Work out the finished part from the listing and answer in its coordinate system (mm). A direction names the side the tool comes from. Round coordinates to 2 decimals unless told otherwise and drop trailing zeros. Loops run counter-clockwise (first coordinate to the right, second up) from the corner with the lowest first, then second, coordinate; pieces in that order, holes last.
```python
from build123d import *

# Parameters (mm, degrees)
SKETCH1_W           = 139
SKETCH1_H           = 62
SKETCH1_R           = 3.75
SKETCH1_R_2         = 1.65
SKETCH1_R_3         = 3.1
SKETCH1_W_2         = 2.2
SKETCH1_H_2         = 1.1
SKETCH1_W_3         = 2.7
SKETCH1_H_3         = 1.2
BOSS_EXTRUDE1_DEPTH = 3


with BuildPart() as part:
    # Sketch1 → Boss-Extrude1 (new body)
    with BuildSketch(Plane.XY):
        with Locations((69.5, 31)):
            Rectangle(SKETCH1_W, SKETCH1_H)
        with Locations((94.5, 10)):
            Circle(SKETCH1_R, mode=Mode.SUBTRACT)
        with Locations((4, 33)):
            Circle(SKETCH1_R_2, mode=Mode.SUBTRACT)
        with Locations((135, 33)):
            Circle(SKETCH1_R_2, mode=Mode.SUBTRACT)
        with Locations((135, 11)):
            Circle(SKETCH1_R_2, mode=Mode.SUBTRACT)
        with Locations((4, 11)):
            Circle(SKETCH1_R_2, mode=Mode.SUBTRACT)
        with Locations((106.75, 31.217622393)):
            Circle(SKETCH1_R, mode=Mode.SUBTRACT)
        with Locations((124, 21.5)):
            Circle(SKETCH1_R_2, mode=Mode.SUBTRACT)
        with Locations((44.5, 10)):
            Circle(SKETCH1_R, mode=Mode.SUBTRACT)
        with Locations(Location((15, 21.5, 0), (0, 0, 180))):
            Circle(SKETCH1_R_2, mode=Mode.SUBTRACT)
        with Locations((56.5, 52)):
            Circle(SKETCH1_R_3, mode=Mode.SUBTRACT)
        with Locations((4, 55)):
            Circle(SKETCH1_R_2, mode=Mode.SUBTRACT)
        with Locations((135, 55)):
            Circle(SKETCH1_R_2, mode=Mode.SUBTRACT)
        with Locations((44.5, 3.75)):
            Rectangle(SKETCH1_W_2, SKETCH1_H_2, mode=Mode.SUBTRACT)
        with Locations((94.5, 3.75)):
            Rectangle(SKETCH1_W_2, SKETCH1_H_2, mode=Mode.SUBTRACT)
        with Locations((106.75, 24.967622393)):
            Rectangle(SKETCH1_W_2, SKETCH1_H_2, mode=Mode.SUBTRACT)
        with Locations((56.5, 46)):
            Rectangle(SKETCH1_W_3, SKETCH1_H_3, mode=Mode.SUBTRACT)
        with BuildLine():
            Line((114.936628972, 47.05), (119.063371028, 47.05))
            ThreePointArc((119.063371028, 47.05), (120.6, 50), (119.063371028, 52.95))
            Line((119.063371028, 52.95), (114.936628972, 52.95))
            ThreePointArc((114.936628972, 52.95), (113.4, 50), (114.936628972, 47.05))
        make_face(mode=Mode.SUBTRACT)
        with BuildLine():
            Line((30.186628972, 28.267622393), (34.313371028, 28.267622393))
            ThreePointArc((34.313371028, 28.267622393), (35.85, 31.217622393), (34.313371028, 34.167622393))
            Line((34.313371028, 34.167622393), (30.186628972, 34.167622393))
            ThreePointArc((30.186628972, 34.167622393), (28.65, 31.217622393), (30.186628972, 28.267622393))
        make_face(mode=Mode.SUBTRACT)
    extrude(amount=BOSS_EXTRUDE1_DEPTH)


solid = part.part
```
1. Which of the six approach directions +Z, -Z, +X, -X, +Y, -Y give full straight-line access (tool end or side, diameter ignored) to faces 5 (the face through (28.65, 31.27, 1.48)), 6 (the face through (69, 0, 1))?
Answer key:
face 5: +Z, -Z
face 6: +Z, -Z, +X, -X, -Y
2. Determine the mould class of faces 1 (the face through (117, 52.95, 1)), 2 (the face through (136.574, 33.496, 1.479)), 3 (the face through (0, 31, 1)), 4 (the face through (69, 62, 1)) for opening direction X: +X half, -X half, draft (parallel to the pull), parting line (faces both ways), or undercut.
Answer key:
face 1: undercut
face 2: undercut
face 3: -X half
face 4: draft
3. Consider probe 1 along Y at (x, z) = (135, 2.2); probe 2 along Y at (x, z) = (44.5, 1.05); probe 3 along Y at (x, z) = (55.5, 1.1). Determine where each line is inside the solid, lowest interval first.
Answer key:
probe 1: y = 0 to 9.35, 12.65 to 31.35, 34.65 to 53.35, 56.65 to 62
probe 2: y = 0 to 3.2, 4.3 to 6.25, 13.75 to 62
probe 3: y = 0 to 45.4, 46.6 to 49.07, 54.93 to 62
4. Given pin 1 (2 mm diameter, centred on x = 135, y = 55, fed in from +Z), flat-ended and moving along its own axis, determine where the tip first touches the part or whether it passes through.
Answer key:
pin 1: passes through
5. Find section C-C (z = 1.7). Give the number of separate pieces and of enclosed holes in the cut face, then the cut area to 3 significant figures.
Answer key:
separate pieces: 1
enclosed holes: 18
area: 8,300 mm2
6. Find section B-B (y = 21.5). Write down the section's boundary in (x, z), then the cut area to 3 significant figures.
Answer key:
outline: (0, 0) - (13.35, 0) - (13.35, 3) - (0, 3) - close; (16.65, 0) - (122.35, 0) - (122.35, 3) - (16.65, 3) - close; (125.65, 0) - (139, 0) - (139, 3) - (125.65, 3) - close
area: 397 mm2
7. Find section A-A (x = 56.5). Write down the section's boundary in (y, z), then the cut area to 3 significant figures.
Answer key:
outline: (0, 0) - (45.4, 0) - (45.4, 3) - (0, 3) - close; (46.6, 0) - (48.9, 0) - (48.9, 3) - (46.6, 3) - close; (55.1, 0) - (62, 0) - (62, 3) - (55.1, 3) - close
area: 164 mm2
